```python
from build123d import *

# Parameters (mm, degrees)
BOSS_EXTRUDE1_DEPTH = 11.5
CUT_EXTRUDE1_DEPTH  = 16.62921943
FILLET1_R           = 0.5


with BuildPart() as part:
    # Sketch1 → Boss-Extrude1 (new, symmetric)
    with BuildSketch(Plane(origin=(0, 0, 0), x_dir=(0, 0, -1), z_dir=(1, 0, 0))):
        Polygon((-10.15, -1.45), (3.75, -1.45), (3.75, 4.45), (-3.75, 4.45), (-3.75, 1.45), (-10.15, 1.45), align=None)
    extrude(amount=BOSS_EXTRUDE1_DEPTH, both=True)

    # Sketch2 → Cut-Extrude1 (cut, through all)
    with BuildSketch(Plane(origin=(0, 1.45, 0), x_dir=(1, 0, 0), z_dir=(0, 1, 0))):
        with BuildLine():
            Line((-8.263922466, -5.6), (-5.736077534, -5.6))
            ThreePointArc((-5.736077534, -5.6), (-5, -7.15), (-5.736077534, -8.7))
            Line((-5.736077534, -8.7), (-8.263922466, -8.7))
            ThreePointArc((-8.263922466, -8.7), (-9, -7.15), (-8.263922466, -5.6))
        make_face()
        with BuildLine():
            Line((5.736077534, -5.6), (8.263922466, -5.6))
            ThreePointArc((8.263922466, -5.6), (9, -7.15), (8.263922466, -8.7))
            Line((8.263922466, -8.7), (5.736077534, -8.7))
            ThreePointArc((5.736077534, -8.7), (5, -7.15), (5.736077534, -5.6))
        make_face()
    extrude(amount=-CUT_EXTRUDE1_DEPTH, mode=Mode.SUBTRACT)

    # Fillet1
    fillet1_edges = [part.edges().sort_by_distance(p)[0] for p in [
        (11.5, 1.5, -3.75),
        (11.5, 2.95, 3.75),
        (-11.5, 2.95, 3.75),
        (-11.5, 1.5, -3.75),
    ]]
    fillet(fillet1_edges, radius=FILLET1_R)


solid = part.part
```
Source: CAD feature listing. Evaluate the final solid. Frame: model axes, mm. A direction names the side the tool comes from. Round coordinates to 2 decimals unless told otherwise and drop trailing zeros. Loops run counter-clockwise (first coordinate to the right, second up) from the corner with the lowest first, then second, coordinate; pieces in that order, holes last. Notation, with made-up numbers: M -5.5,89 L 31.5,89 A26 ccw 31.5,112 Z; hole C -32.75,-30 d4. An arc over 180 degrees is marked long. Use a Markdown table: item, result. Add a question column.
1. Section query B-B on y = 0.45. Return the cut outline in (x, z), then the cut area to 3 significant figures.
2. Section query A-A on x = 7.5. Return the cut outline in (y, z), then the cut area to 3 significant figures.
3. Section query D-D on y = 1.9. Return the cut outline in (x, z).
4. Mould query, pull axis Z, two halves, no side actions, for faces 3 (the flat face through (0, 4.45, 0)), 4 (the cylindrical face through (-5, 0, 7.1)), 5 (the flat face through (0, 3, 3.75)). Classes: pulls with the +Z half, pulls with the -Z half, needs draft (parallel to the pull), parting line crosses it, or undercut.
5. Reachability of faces 1 (the flat face through (-7, 0, 5.6)), 2 (the flat face through (0, 1, -3.75)) from +Z, -Z, +X, -X, +Y, -Y: full face, straight path, thin tool, end or side. Return the list, or none.
6. Section query C-C on z = 6. Return the cut outline in (x, y), then the cut area to 3 significant figures.
7. Line query: line 1 (Z direction, x = -7.75, y = 0.6); line 2 (Y direction, x = 9, z = 8.25); line 3 (Z direction, x = 3.25, y = 2.2). Output: solid intervals per line, ascending.
8. Contact query for flat-ended pins moving along their axis: P1, Ø0.9, axis at x = -1.5, y = 3, coming from the +Z side; P2, Ø1.5, axis at x = 3.5, z = 7.5, coming from the +Y side. Output: stop coordinate, or through.
Reported:
| question | item | result |
|---|---|---|
| 1 | outline | M -11.5,-3.25 A0.5 ccw -11,-3.75 L 11,-3.75 A0.5 ccw 11.5,-3.25 L 11.5,10.15 L -11.5,10.15 Z; hole M -8.26,5.6 L -5.74,5.6 A2 ccw -5.74,8.7 L -8.26,8.7 A2 ccw Z; hole M 5.74,5.6 L 8.26,5.6 A2 ccw 8.26,8.7 L 5.74,8.7 A2 ccw Z |
| 1 | area | 298 mm² |
| 2 | outline | M -1.45,-3.75 L 4.45,-3.75 L 4.45,3.75 L 1.45,3.75 L 1.45,5.6 L -1.45,5.6 Z; M -1.45,8.7 L 1.45,8.7 L 1.45,10.15 L -1.45,10.15 Z |
| 2 | area | 53.8 mm² |
| 3 | outline | M -11.5,-3.25 A0.5 ccw -11,-3.75 L 11,-3.75 A0.5 ccw 11.5,-3.25 L 11.5,3.25 A0.5 ccw 11,3.75 L -11,3.75 A0.5 ccw -11.5,3.25 Z |
| 4 | face 3 | needs draft |
| 4 | face 4 | undercut |
| 4 | face 5 | pulls with the +Z half |
| 5 | face 1 | +Y, -Y |
| 5 | face 2 | -Z, +X, -X, +Y, -Y |
| 6 | outline | M -11.5,-1.45 L -8.64,-1.45 L -8.64,1.45 L -11.5,1.45 Z; M -5.36,-1.45 L 5.36,-1.45 L 5.36,1.45 L -5.36,1.45 Z; M 8.64,-1.45 L 11.5,-1.45 L 11.5,1.45 L 8.64,1.45 Z |
| 6 | area | 47.7 mm² |
| 7 | line 1 | z = -3.75 to 5.6, 8.7 to 10.15 |
| 7 | line 2 | y = -1.45 to 1.45 |
| 7 | line 3 | z = -3.75 to 3.75 |
| 8 | P1 | stops at z = 3.75 |
| 8 | P2 | stops at y = 1.45 |
